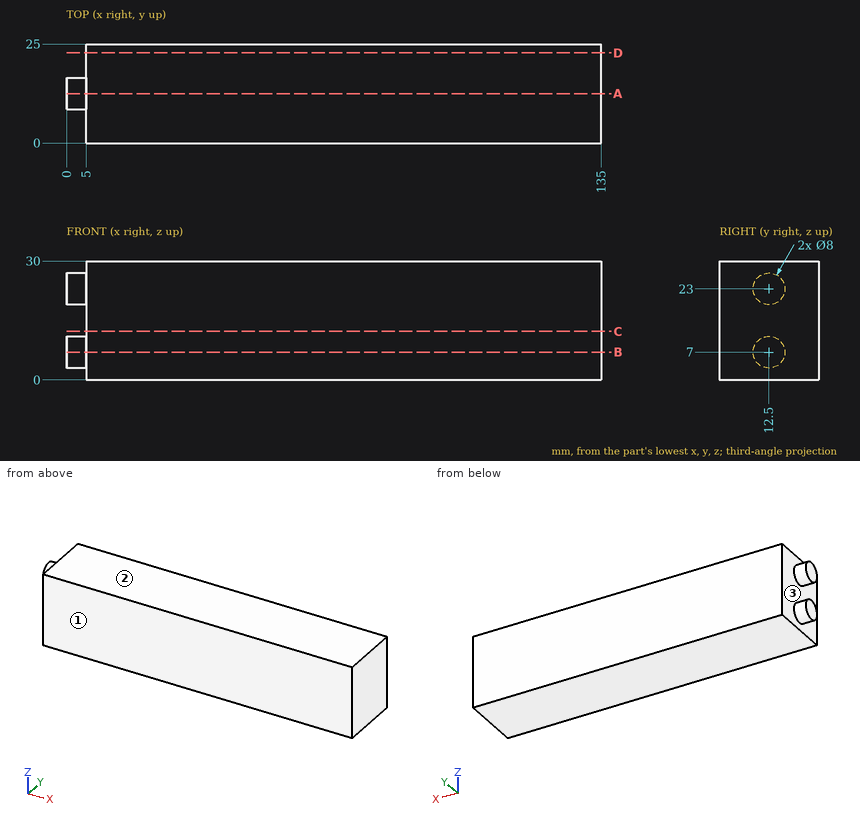
Can you work these out from the drawing? Everything is in mm from the part's minimum corner. Round coordinates to 2 decimals unless told otherwise and drop trailing zeros. Order: outer loops, then holes, each group sorted by start corner. A loop starts at its lowest first (then second) coordinate and runs counter-clockwise, first axis right, second up. Notation, with made-up numbers: (29.25, 50.25) -> (61.25, 50.25) arc R11 ccw to (61.25, 56.25) -> close; hole circle Ø1 at (61.25, -7). An arc over 180 degrees is marked (long way). Return JSON: item names as keys, results as strings. Group by question number.
1. Will this pin go through, and if not, where does the flat tip stop? pin 1 (2 mm diameter, centred on y = 6.5, z = 3.5, fed in from -X).
2. I need wall thicknesses on line 1 (X direction, y = 15.25, z = 12.5). Which ranges of the line are inside material? Lowest first, please. Write a range as [from, to].
3. We'd pull the mould along Z, two halves only. Please class the marked faces 1, 2 and 3: released by +Z, released by -Z, zero draft, split by the parting line, or undercut.
4. If we section it at D-D, the plane y = 22.75: Write out the boundary of the cut face in (x, z).
5. If we section it at A-A, the plane y = 12.5: Write out the boundary of the cut face in (x, z), then the cut area to 3 significant figures.
6. If we section it at B-B, the plane z = 7: Write out the boundary of the cut face in (x, y), then the cut area to 3 significant figures.
7. If we section it at C-C, the plane z = 12.25: Write out the boundary of the cut face in (x, y), then the cut area to 3 significant figures.
Output values:
{
 "1": {"pin 1": "x = 5"},
 "2": {"line 1": "[5, 135]"},
 "3": {"face 1": "zero draft", "face 2": "released by +Z", "face 3": "undercut"},
 "4": {"outline": "(5, 0) -> (135, 0) -> (135, 30) -> (5, 30) -> close"},
 "5": {"outline": "(0, 3) -> (5, 3) -> (5, 0) -> (135, 0) -> (135, 30) -> (5, 30) -> (5, 27) -> (0, 27) -> (0, 19) -> (5, 19) -> (5, 11) -> (0, 11) -> close", "area": "3,980 mm²"},
 "6": {"outline": "(0, 8.5) -> (5, 8.5) -> (5, 0) -> (135, 0) -> (135, 25) -> (5, 25) -> (5, 16.5) -> (0, 16.5) -> close", "area": "3,290 mm²"},
 "7": {"outline": "(5, 0) -> (135, 0) -> (135, 25) -> (5, 25) -> close", "area": "3,250 mm²"}
}
